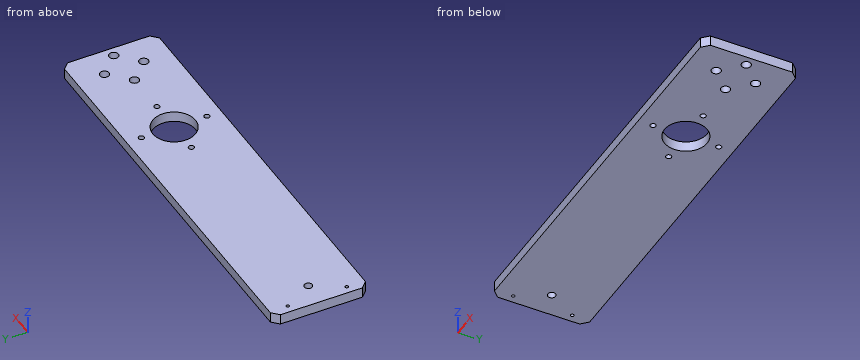
from build123d import *

# Parameters (mm, degrees)
SKETCH_1_R              = 7
SKETCH_1_R_2            = 3
SKETCH_1_R_3            = 32.5
EXTRUDE_1_DEPTH         = 16
HOLE_WIZARD_M14_1_D     = 12
HOLE_WIZARD_M14_1_DEPTH = 34
HOLE_WIZARD_M14_1_TIP   = 3.605163714
HOLE_WIZARD_M6_1_D      = 5
HOLE_WIZARD_M6_1_DEPTH  = 18
HOLE_WIZARD_M6_1_TIP    = 1.502151548
HOLE_WIZARD_M10_2_D     = 8.5
HOLE_WIZARD_M10_2_DEPTH = 24.5
HOLE_WIZARD_M10_2_TIP   = 2.553657631


with BuildPart() as part:
    # 草图1 → 凸台-拉伸1 (new body)
    with BuildSketch(Plane.XY):
        Polygon((637.687566056, 879.677968159), (637.687566056, 754.677968159), (647.687566056, 744.677968159), (1244.687566056, 744.677968159), (1254.687566056, 754.677968159), (1254.687566056, 879.677968159), (1244.687566056, 889.677968159), (647.687566056, 889.677968159), align=None)
        with Locations((1209.687566056, 787.177968159)):
            Circle(SKETCH_1_R, mode=Mode.SUBTRACT)
        with Locations((1064.687566056, 767.177968159)):
            Circle(SKETCH_1_R_2, mode=Mode.SUBTRACT)
        with Locations((1064.687566056, 817.177968159)):
            Circle(SKETCH_1_R_3, mode=Mode.SUBTRACT)
        with Locations((1014.687566056, 817.177968159)):
            Circle(SKETCH_1_R_2, mode=Mode.SUBTRACT)
        with Locations((1114.687566056, 817.177968159)):
            Circle(SKETCH_1_R_2, mode=Mode.SUBTRACT)
        with Locations((1064.687566056, 867.177968159)):
            Circle(SKETCH_1_R_2, mode=Mode.SUBTRACT)
        with Locations((1239.687566056, 817.177968159)):
            Circle(SKETCH_1_R, mode=Mode.SUBTRACT)
        with Locations((1179.687566056, 817.177968159)):
            Circle(SKETCH_1_R, mode=Mode.SUBTRACT)
        with Locations((1209.687566056, 847.177968159)):
            Circle(SKETCH_1_R, mode=Mode.SUBTRACT)
    extrude(amount=EXTRUDE_1_DEPTH)

    # M14 螺纹孔1
    with Locations(Plane.XY.offset(16)):
        with Locations((675.687566056, 817.177968159)):
            Hole(HOLE_WIZARD_M14_1_D / 2, depth=HOLE_WIZARD_M14_1_DEPTH)
            with Locations((0, 0, -(HOLE_WIZARD_M14_1_DEPTH + HOLE_WIZARD_M14_1_TIP / 2))):  # 118° drill point
                Cone(0, HOLE_WIZARD_M14_1_D / 2, HOLE_WIZARD_M14_1_TIP, mode=Mode.SUBTRACT)

    # M6 螺纹孔1
    with Locations(Plane(origin=(0, 0, 0), x_dir=(-1, 0, 0), z_dir=(0, 0, -1))):
        with Locations((-649.687566056, 772.177968159), (-649.687566056, 862.177968159)):
            Hole(HOLE_WIZARD_M6_1_D / 2, depth=HOLE_WIZARD_M6_1_DEPTH)
            with Locations((0, 0, -(HOLE_WIZARD_M6_1_DEPTH + HOLE_WIZARD_M6_1_TIP / 2))):  # 118° drill point
                Cone(0, HOLE_WIZARD_M6_1_D / 2, HOLE_WIZARD_M6_1_TIP, mode=Mode.SUBTRACT)

    # M10 螺纹孔2
    with Locations(Plane.XY.offset(16)):
        with Locations((1014.687566056, 817.177968159), (1064.687566056, 767.177968159), (1114.687566056, 817.177968159), (1064.687566056, 867.177968159)):
            Hole(HOLE_WIZARD_M10_2_D / 2, depth=HOLE_WIZARD_M10_2_DEPTH)
            with Locations((0, 0, -(HOLE_WIZARD_M10_2_DEPTH + HOLE_WIZARD_M10_2_TIP / 2))):  # 118° drill point
                Cone(0, HOLE_WIZARD_M10_2_D / 2, HOLE_WIZARD_M10_2_TIP, mode=Mode.SUBTRACT)


solid = part.part
Could you check a few things on this model? Use its own coordinates, in mm. Coordinates: 2 decimals unless noted, no trailing zeros. Order: outer loops, then holes, each group sorted by start corner. A loop starts at its lowest first (then second) coordinate and runs counter-clockwise, first axis right, second up.
Q1. Please list where these lines run through material, in increasing order: L1, parallel to X at y = 867, z = 14.5; L2, parallel to Y at x = 1042, z = 9; L3, parallel to X at y = 784.5, z = 2.75.
Q2. Suppose I cut it at A-A on z = 6. Give the number of separate pieces and of enclosed holes in the cut face, and give its area (3 significant figures).
Q3. Suppose I cut it at B-B on x = 1052. Please give me the cut outline in (y, z).
Answer:
1. L1: x = 637.69 to 1060.44, 1068.93 to 1254.69
1. L2: y = 744.68 to 793.91, 840.45 to 889.68
1. L3: x = 637.69 to 1203.22, 1216.16 to 1254.69
2. separate pieces: 1
2. enclosed holes: 12
2. area: 85,000 mm2
3. outline: (744.68, 0) - (787.26, 0) - (787.26, 16) - (744.68, 16) - close; (847.1, 0) - (889.68, 0) - (889.68, 16) - (847.1, 16) - close
